CAD build for the part. Positions are in the model's coordinates, mm. A direction names the side the tool comes from. Give positions to 0.01 mm unless a question says otherwise; leave off trailing zeros. Write each loop counter-clockwise with the first axis right and the second up, starting at its lowest first coordinate (ties: lowest second). Pieces come first, ordered by that corner, then holes. Notation, with made-up numbers: (-38, 16) - (11, 16) arc R25 cw to (11, 31) - close; hole circle Ø5 at (16.25, 62). An arc over 180 degrees is marked (long way). Answer as a JSON object with one key per item and string values.
from build123d import *

# Parameters (mm, degrees)
BOSS_EXTRUDE1_DEPTH = 4
SKETCH2_R           = 3
CUT_EXTRUDE1_DEPTH  = 42.424630354
BOSS_EXTRUDE2_DEPTH = 4
SKETCH3_R           = 2.6
CUT_EXTRUDE2_DEPTH  = 60.58873158
SKETCH4_OUTSIDE_W   = 38.8
SKETCH4_OUTSIDE_H   = 34.8
CUT_EXTRUDE3_DEPTH  = 16.522711642


with BuildPart() as part:
    # Sketch1 → Boss-Extrude1 (new body)
    with BuildSketch(Plane(origin=(0, 0, 0), x_dir=(1, 0, 0), z_dir=(0, 1, 0))):
        with BuildLine():
            Line((-30, 10), (30, 10))
            ThreePointArc((30, 10), (40, 0), (30, -10))
            Line((30, -10), (-30, -10))
            ThreePointArc((-30, -10), (-40, 0), (-30, 10))
        make_face()
    extrude(amount=BOSS_EXTRUDE1_DEPTH)

    # Sketch2 → Cut-Extrude1 (cut, through all)
    with BuildSketch(Plane(origin=(0, 4, 0), x_dir=(1, 0, 0), z_dir=(0, 1, 0))):
        with Locations(Location((-30, 0, 0), (0, 0, 270))):
            Circle(SKETCH2_R)
        with Locations(Location((30, 0, 0), (0, 0, 270))):
            Circle(SKETCH2_R)
    extrude(amount=-CUT_EXTRUDE1_DEPTH, mode=Mode.SUBTRACT)

    # 3DSketch1 → Boss-Extrude2 (add)
    with BuildSketch(Plane(origin=(-16.522711642, 4, 10), x_dir=(0, 0.447213595499958, -0.894427190999916), z_dir=(-1, 0, 0))):
        with BuildLine():
            Line((0, 0), (10.733126292, 5.366563146))
            Line((10.733126292, 5.366563146), (13.416407865, 0))
            ThreePointArc((13.416407865, 0), (10.733126292, -8.049844719), (2.683281573, -5.366563146))
            Line((2.683281573, -5.366563146), (0, 0))
        make_face()
    boss_extrude2 = extrude(amount=BOSS_EXTRUDE2_DEPTH)

    # Sketch3 → Cut-Extrude2 (cut, through all)
    with BuildSketch(Plane(origin=(-16.522711642, 0, 0), x_dir=(0, 0, -1), z_dir=(1, 0, 0))):
        with Locations((-4, 10)):
            Circle(SKETCH3_R)
    cut_extrude2 = extrude(amount=-CUT_EXTRUDE2_DEPTH, mode=Mode.SUBTRACT)

    # Sketch4 outside → Cut-Extrude3 (cut)
    with BuildSketch(Plane(origin=(0, 0, 0), x_dir=(0, 0, -1), z_dir=(1, 0, 0))):
        with Locations((0, 8)):
            Rectangle(SKETCH4_OUTSIDE_W, SKETCH4_OUTSIDE_H)
        Polygon((-10, 2), (-2.3, 2), (10, 0.5), (10, 0), (-10, 0), align=None, mode=Mode.SUBTRACT)
    cut_extrude3 = extrude(amount=-CUT_EXTRUDE3_DEPTH, mode=Mode.SUBTRACT)

    # Mirror1: Boss-Extrude2, Cut-Extrude2, Cut-Extrude3 across plane
    add(boss_extrude2.mirror(Plane(origin=(0, 0, 0), x_dir=(0, 0, 1), z_dir=(1, 0, 0))))
    add(cut_extrude2.mirror(Plane(origin=(0, 0, 0), x_dir=(0, 0, 1), z_dir=(1, 0, 0))), mode=Mode.SUBTRACT)
    add(cut_extrude3.mirror(Plane(origin=(0, 0, 0), x_dir=(0, 0, 1), z_dir=(1, 0, 0))), mode=Mode.SUBTRACT)


solid = part.part
Item 1: Cut at A-A (z = -0.5). Give the cut face in (x, y), and give its area (3 significant figures).
Entries:
{"outline": "(-39.99, 0) - (-32.96, 0) - (-32.96, 4) - (-39.99, 4) - close; (-27.04, 0) - (27.04, 0) - (27.04, 4) - (20.52, 4) - (20.52, 13.97) - (16.52, 13.97) - (16.52, 1.66) - (-16.52, 1.66) - (-16.52, 13.97) - (-20.52, 13.97) - (-20.52, 4) - (-27.04, 4) - close; (32.96, 0) - (39.99, 0) - (39.99, 4) - (32.96, 4) - close", "area": "275 mm2"}
Item 2: Cut at D-D (z = -7). Give the cut face in (x, y).
Entries:
{"outline": "(-37.14, 0) - (37.14, 0) - (37.14, 4) - (16.52, 4) - (16.52, 0.87) - (-16.52, 0.87) - (-16.52, 4) - (-37.14, 4) - close"}
Item 3: Cut at B-B (x = -28). Give the cut face in (y, z), and give its area (3 significant figures).
Entries:
{"outline": "(0, -10) - (4, -10) - (4, -2.24) - (0, -2.24) - close; (0, 2.24) - (4, 2.24) - (4, 10) - (0, 10) - close", "area": "62.1 mm2"}
Item 4: Mould opens along X. For faces 6 (the cylindrical face through (-29.1, 2.03, 2.86)), 7 (the cylindrical face through (18.49, 7.46, 4.56)), 8 (the flat face through (-20.523, 7, 4)) say: +X half, -X half, draft (parallel to the pull), parting line (faces both ways), or undercut.
Entries:
{"face 6": "undercut", "face 7": "draft", "face 8": "-X half"}
Item 5: Cut at C-C (x = 24). Give the cut face in (y, z), and give its area (3 significant figures).
Entries:
{"outline": "(0, -10) - (4, -10) - (4, 10) - (0, 10) - close", "area": "80.0 mm2"}
Item 6: Flat gauge pins, fed straight in: P1, Ø6, axis at y = 9.5, z = 5, coming from the -X side; P2, Ø6, axis at x = -25.5, z = -4.5, coming from the +Y side; P3, Ø7, axis at y = 10, z = 4, coming from the +X side. Where does each tip first touch, or does it go through?
Entries:
{"P1": "x = -20.52", "P2": "y = 4", "P3": "x = 20.52"}
Item 7: Probe line 1 (X direction, y = 2.1, z = 0); line 2 (X direction, y = 1.6, z = 0); line 3 (Y direction, x = 17.9, z = 4). List the from-to ranges inside material, lowest first. Write a range as from..to.
Entries:
{"line 1": "-40..-33, -27..-16.52, 16.52..27, 33..40", "line 2": "-40..-33, -27..27, 33..40", "line 3": "0..7.4, 12.6..16"}
Item 8: Which spindle directions (+Z, -Z, +X, -X, +Y, -Y) get a long thin tool onto all of the face, cutting with end or side? Do faces 1 (the flat face through (-18, 7, -2)), 2 (the cylindrical face through (-18.49, 7.46, 4.56)), 3 (the flat face through (0.23, 1.26, -3.76)), 4 (the flat face through (20.523, 7, 4)), 5 (the flat face through (0.4, 1.6, 10)). Say none if no direction does.
Entries:
{"face 1": "-Z, +X, -X, +Y", "face 2": "+X, -X", "face 3": "-Z, +Y", "face 4": "+Z, -Z, +X, +Y", "face 5": "+Z, +X, -X, +Y, -Y"}
